Design review of the part built by this model. Coordinates are the model's own, in mm. Face numbers are marked on the shaded views. A direction names the side the tool comes from. Round coordinates to 2 decimals unless told otherwise and drop trailing zeros. Order: outer loops, then holes, each group sorted by start corner. A loop starts at its lowest first (then second) coordinate and runs counter-clockwise, first axis right, second up.
Autodesk Inventor part; units mm, degrees
ref_plane "Work Plane1" through (1.525, 0, 0) normal (0, 0, 1) x (1, 0, 0)
ref_plane "YZ Plane" through (0, 0, 0) normal (1, 0, 0) x (0, 1, 0)
ref_plane "XZ Plane" through (0, 0, 0) normal (0, 1, 0) x (-1, 0, 0)
sketch "Sketch1" plane through (0, 0, 0) normal (0, 0, 1) x (1, 0, 0)
  line L0 (0, 4) -> (0, 2.5)
  line L1 (34, 2.5) -> (50, 2.5)
  line L2 (50, 2.5) -> (50, 0)
  line L3 (50, 0) -> (-0.5001, 0)
  line L4 (-10.6001, 0) -> (60.1, 0)
  line L5 (-0.5001, 0) -> (-0.5001, 4)
  line L6 (-0.5001, 4) -> (0, 4)
  line L7 (34, 2.5) -> (33.5091, 2.5)
  line L8 (33.5091, 2.5) -> (0, 2.5)
  line L9 (0, -0.8) -> (0, 4.8)
  dimension "d0" = 50
  dimension "d1" = 16
  dimension "d2" = 5
  dimension "d9" = 0.5001
  dimension "d10" = 8
  dimension "d13" = 0.4909
  dimension "d14" = 5
revolve "Body" add sketch "Sketch1" angle 360 about axis through (50, 0, 0) along (-1, 0, 0)
sketch "Sketch2" plane through (-0.5001, 0, 0) normal (-1, 0, 0) x (0, 0, 1)
  line L0 (0, 4.6188) -> (4, 2.3094)
  line L1 (4, 2.3094) -> (4, -2.3094)
  line L2 (4, -2.3094) -> (0, -4.6188)
  line L3 (0, -4.6188) -> (-4, -2.3094)
  line L4 (-4, -2.3094) -> (-4, 2.3094)
  line L5 (-4, 2.3094) -> (0, 4.6188)
  point P0 (0, 0)
  point P1 (0, 0)
  dimension "d11" = 8
extrude "Head" add sketch "Sketch2" along normal blind 3.38
sketch "Sketch4" plane through (0, 0, 0) normal (0, 0, 1) x (1, 0, 0)
  line L0 (-3.8801, 4) -> (-3.8801, 4.6188)
  line L1 (-3.8801, 4.6188) -> (-3.5228, 4.6188)
  line L2 (-3.5228, 4.6188) -> (-3.8801, 4)
  line L3 (-4.5561, 0) -> (0.1759, 0)
  line L4 (-0.5001, 4.6188) -> (-3.8801, 4.6188)
  line L5 (-3.8801, 2.3094) -> (-3.8801, 4.6188)
  dimension "d5" = 30
  dimension "d19" = 8
revolve "Chamfer1" cut sketch "Sketch4" angle 360 about axis through (-10, 0, 0) along (1, 0, 0)
thread "Thread"
chamfer "Chamfer2" distance 0.4908 distance2 0.4909 1 edges at (50, -2.5, 0) measured on face at (50, -0.2955, -1.5537)
ref_plane "Work Plane1" through (1.525, 0, 0) normal (0, 0, 1) x (1, 0, 0)
equation "\"d0\" = NLG"
equation "\"d1\" = GEL"
equation "\"d2\" = GD"
equation "\"d10\" = SD2"
equation "\"d14\" = BDM"
equation "\"d11\" = SW"
equation "\"d3\" = KOH - SD"
equation "\"d5\" = ANG1"
equation "\"d19\" = SW0"
equation "\"d15\" = GEL"
equation "\"d6\" = -0.5 * SPD + 0.5 * GD"
equation "\"NLG\" = 50"
equation "\"GD\" = NND"
equation "\"BDM\" = NND"
equation "\"KOH\" = 3.88"
equation "\"GEL\" = 16"
equation "\"SW\" = 8"
equation "\"SW0\" = SW"
equation "\"SPD\" = NND - 1.2269 * PTC"
equation "\"SD2\" = SW"
equation "\"SD\" = 0.5"
equation "\"ANG1\" = 30deg"
equation "\"GAL\" = 0.61345 * PTC"
equation "\"GUL\" = 0.61345 * PTC"
equation "\"RR\" = 0.2"
equation "\"WFT\" = SD"
equation "\"GD1\" = THREADDIA - 1.2269 * PTC"
equation "\"THREADDIA\" = 5"
equation "\"SDH\" = SW"
equation "\"TOA\" = 30deg"
equation "\"FAWI\" = 45deg"
equation "\"PTC\" = 0.8"
equation "\"NND\" = 5"
equation "\"E0\" = 1.155 * SW"
properties part number "AS 1111 - M5 x 50" material "Steel, Mild"
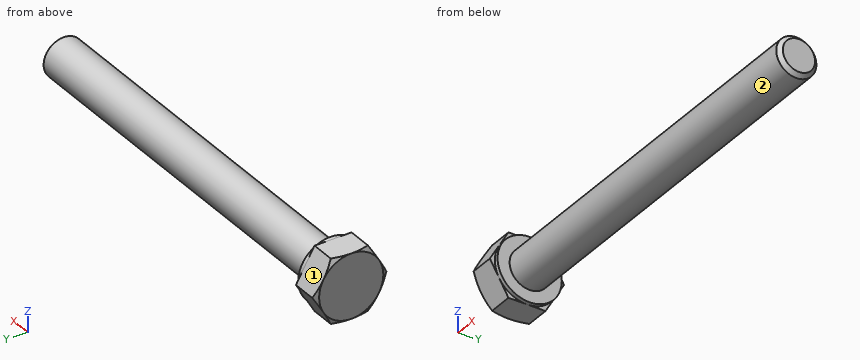
1) Clearance check with flat-ended pins moving along their axes: P1, Ø1.6, axis at y = -1.5, z = -2.5, coming from the +X side; P2, Ø0.9, axis at y = -4, z = 0.5, coming from the +X side; P3, Ø1.5, axis at x = 30.5, y = 2, coming from the +Z side. State where each tip first meets the part, or that it passes through.
Results:
P1: stops at x = 49.89
P2: stops at x = 0
P3: stops at z = 2.17
2) For the marked faces 1 and 2, list the 3-axis set-ups (+Z, -Z, +X, -X, +Y, -Y) from which the entire face can be reached by the end or side of a thin tool; tool diameter is ignored.
Results:
face 1: +Z, +X, -X, +Y
face 2: +X
3) Take a section at A-A on x = 3. Give the boundary of the cut face in (y, z).
Results:
outline: circle Ø5 at (0, 0)
4) To check wall thickness, follow line 1 along X through (y, z) = (2, -2.75); line 2 along Z through (x, y) = (10, 1.5); line 3 along Y through (x, z) = (37, 0.75). State the ranges of each line that lie inside material, in increasing order.
Results:
line 1: x = -3.88 to 0
line 2: z = -2 to 2
line 3: y = -2.38 to 2.38
